Source: CAD feature listing. Evaluate the final solid. Frame: model axes, mm. A direction names the side the tool comes from. Give positions to 0.01 mm unless a question says otherwise; leave off trailing zeros. Order: outer loops, then holes, each group sorted by start corner. A loop starts at its lowest first (then second) coordinate and runs counter-clockwise, first axis right, second up. Notation, with made-up numbers: (-2.5, -30) -> (21.5, -30) arc R10 ccw to (21.5, -20) -> close; hole circle Ø1 at (86, 86.5). An arc over 180 degrees is marked (long way). Answer in a Markdown table with one row per item.
```python
from build123d import *

# Parameters (mm, degrees)
BOSS_EXTRUDE1_DEPTH = 60.3
SKETCH2_W           = 20.9
SKETCH2_H           = 8.4
BOSS_EXTRUDE2_DEPTH = 4.55
FILLET1_R           = 1
CHAMFER1_SIZE       = 0.5


with BuildPart() as part:
    # Sketch1 → Boss-Extrude1 (new body)
    with BuildSketch(Plane(origin=(0, 0, 0), x_dir=(1, 0, 0), z_dir=(0, 1, 0))):
        with BuildLine():
            Line((-7.8, 3.05), (7.8, 3.05))
            ThreePointArc((7.8, 3.05), (9.214213562, 2.464213562), (9.8, 1.05))
            Line((9.8, 1.05), (9.8, -1.05))
            ThreePointArc((9.8, -1.05), (9.214213562, -2.464213562), (7.8, -3.05))
            Line((7.8, -3.05), (-7.8, -3.05))
            ThreePointArc((-7.8, -3.05), (-9.214213562, -2.464213562), (-9.8, -1.05))
            Line((-9.8, -1.05), (-9.8, 1.05))
            ThreePointArc((-9.8, 1.05), (-9.214213562, 2.464213562), (-7.8, 3.05))
        make_face()
    extrude(amount=BOSS_EXTRUDE1_DEPTH)

    # Sketch2 → Boss-Extrude2 (add)
    with BuildSketch(Plane(origin=(0, 0, 0), x_dir=(1, 0, 0), z_dir=(0, 1, 0))):
        Rectangle(SKETCH2_W, SKETCH2_H)
    extrude(amount=-BOSS_EXTRUDE2_DEPTH)

    # Fillet1
    fillet1_edges = [part.edges().sort_by_distance(p)[0] for p in [
        (9.214213562, 60.3, -2.464213562),
        (0, 60.3, -3.05),
        (-9.214213562, 60.3, -2.464213562),
        (-9.8, 60.3, 0),
        (-9.214213562, 60.3, 2.464213562),
        (0, 60.3, 3.05),
        (9.214213562, 60.3, 2.464213562),
        (9.8, 60.3, 0),
    ]]
    fillet(fillet1_edges, radius=FILLET1_R)

    # Chamfer1
    chamfer1_edges = [part.edges().sort_by_distance(p)[0] for p in [
        (10.45, -4.55, 0),
        (0, -4.55, 4.2),
        (-10.45, -4.55, 0),
        (0, -4.55, -4.2),
    ]]
    chamfer(chamfer1_edges, length=CHAMFER1_SIZE)


solid = part.part
```
(1) Section query B-B (y = 41). Return the cut outline in (x, z).
A:
| item | result |
|---|---|
| outline | (-9.8, -1.05) arc R2 ccw to (-7.8, -3.05) -> (7.8, -3.05) arc R2 ccw to (9.8, -1.05) -> (9.8, 1.05) arc R2 ccw to (7.8, 3.05) -> (-7.8, 3.05) arc R2 ccw to (-9.8, 1.05) -> close |
(2) Ray query, probe 1 along Z at (x, y) = (-0.75, 45); probe 2 along Y at (x, z) = (-5.5, -3.25). Return the intervals inside material, ascending.
A:
| item | result |
|---|---|
| probe 1 | z = -3.05 to 3.05 |
| probe 2 | y = -4.55 to 0 |
(3) Section query C-C (z = 0). Return the cut outline in (x, y), plus the area to 3 significant figures.
A:
| item | result |
|---|---|
| outline | (-10.45, -4.05) -> (-9.95, -4.55) -> (9.95, -4.55) -> (10.45, -4.05) -> (10.45, 0) -> (9.8, 0) -> (9.8, 59.3) arc R1 ccw to (8.8, 60.3) -> (-8.8, 60.3) arc R1 ccw to (-9.8, 59.3) -> (-9.8, 0) -> (-10.45, 0) -> close |
| area | 1,280 mm^2 |
(4) First-contact query: pin 1 Ø1.7 at (y, z) = (24, 0) entering from +X; pin 2 Ø2 at (x, y) = (-1, 30) entering from -Z; pin 3 Ø2 at (x, y) = (4.5, 3) entering from +Z. Flat tips, straight axial feed; report the tip coordinate or a pass-through.
A:
| item | result |
|---|---|
| pin 1 | stops at x = 9.8 |
| pin 2 | stops at z = -3.05 |
| pin 3 | stops at z = 3.05 |
(5) Section query A-A (x = 1). Return the cut outline in (y, z), plus the area to 3 significant figures.
A:
| item | result |
|---|---|
| outline | (-4.55, -3.7) -> (-4.05, -4.2) -> (0, -4.2) -> (0, -3.05) -> (59.3, -3.05) arc R1 ccw to (60.3, -2.05) -> (60.3, 2.05) arc R1 ccw to (59.3, 3.05) -> (0, 3.05) -> (0, 4.2) -> (-4.05, 4.2) -> (-4.55, 3.7) -> close |
| area | 405 mm^2 |
(6) Access query for faces 1 (the flat face through (9.8, 29, 0)), 2 (the flat face through (0, 29, -3.05)), 3 (the flat face through (0, 29, 3.05)). Directions: +Z, -Z, +X, -X, +Y, -Y. A direction counts if a zero-diameter tool reaches every point of the face in a straight line with its end or side. Return the directions, or none.
A:
| item | result |
|---|---|
| face 1 | +Z, -Z, +X, +Y |
| face 2 | -Z, +X, -X, +Y |
| face 3 | +Z, +X, -X, +Y |
